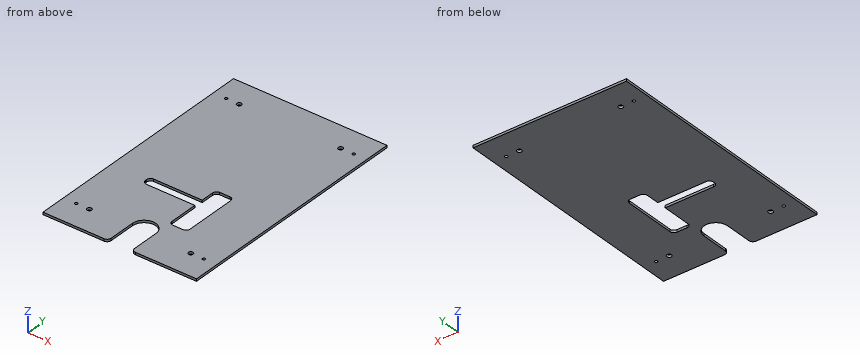
from build123d import *

# Parameters (mm, degrees)
ESQUISSE1_W             = 196
ESQUISSE1_H             = 309
ESQUISSE1_R             = 1.75
ESQUISSE1_R_2           = 3
BOSS_EXTRU_1_DEPTH      = 3
ENL_V_MAT_EXTRU_1_REACH = 5
CONG_1_R                = 5
ENL_V_MAT_EXTRU_2_DEPTH = 4
CONG_2_R                = 5


with BuildPart() as part:
    # Esquisse1 → Boss.-Extru.1 (new body)
    with BuildSketch(Plane.XY):
        Rectangle(ESQUISSE1_W, ESQUISSE1_H)
        with Locations((-81.5, 121.5)):
            Circle(ESQUISSE1_R, mode=Mode.SUBTRACT)
        with Locations((81.5, 121.5)):
            Circle(ESQUISSE1_R, mode=Mode.SUBTRACT)
        with Locations((81.5, -121.5)):
            Circle(ESQUISSE1_R, mode=Mode.SUBTRACT)
        with Locations((-81.5, -121.5)):
            Circle(ESQUISSE1_R, mode=Mode.SUBTRACT)
        with Locations((64.75, 121.5)):
            Circle(ESQUISSE1_R_2, mode=Mode.SUBTRACT)
        with Locations((-64.75, 121.5)):
            Circle(ESQUISSE1_R_2, mode=Mode.SUBTRACT)
        with Locations((-64.75, -121.5)):
            Circle(ESQUISSE1_R_2, mode=Mode.SUBTRACT)
        with Locations((64.75, -121.5)):
            Circle(ESQUISSE1_R_2, mode=Mode.SUBTRACT)
    extrude(amount=BOSS_EXTRU_1_DEPTH)

    # Esquisse2 → Enlèv. mat.-Extru.1 (cut, up to next)
    with BuildSketch(Plane.XY.offset(3), mode=Mode.PRIVATE) as enl_v_mat_extru_1_sk1:
        with BuildLine():
            Line((-15, -154.5), (-15, -115))
            ThreePointArc((-15, -115), (0, -100), (15, -115))
            Line((15, -115), (15, -154.5))
            ThreePointArc((15, -154.5), (0, -169.5), (-15, -154.5))
        make_face()
    enl_v_mat_extru_1_tool1 = extrude(enl_v_mat_extru_1_sk1.sketch, amount=-ENL_V_MAT_EXTRU_1_REACH, mode=Mode.PRIVATE) & part.part
    add(enl_v_mat_extru_1_tool1.solids().sort_by_distance((0, -134.75, 3))[0], mode=Mode.SUBTRACT)

    # Congé1
    cong_1_edges = [part.edges().sort_by_distance(p)[0] for p in [
        (-15, -154.5, 1.5),
        (15, -154.5, 1.5),
    ]]
    fillet(cong_1_edges, radius=CONG_1_R)

    # Esquisse3 → Enlèv. mat.-Extru.2 (cut, through all)
    with BuildSketch(Plane.XY.offset(3)):
        Polygon((-53, -38.5), (14, -38.5), (14, -16.5), (37, -16.5), (37, -92.5), (14, -92.5), (14, -50.5), (-53, -50.5), align=None)
    extrude(amount=-ENL_V_MAT_EXTRU_2_DEPTH, mode=Mode.SUBTRACT)

    # Congé2
    cong_2_edges = [part.edges().sort_by_distance(p)[0] for p in [
        (-53, -50.5, 1.5),
        (-53, -38.5, 1.5),
        (14, -16.5, 1.5),
        (37, -16.5, 1.5),
        (37, -92.5, 1.5),
        (14, -92.5, 1.5),
    ]]
    fillet(cong_2_edges, radius=CONG_2_R)


solid = part.part
The listing builds one solid part. Answer for the finished solid, in the listing's coordinates (mm). Round coordinates to 2 decimals unless told otherwise and drop trailing zeros. Order: outer loops, then holes, each group sorted by start corner. A loop starts at its lowest first (then second) coordinate and runs counter-clockwise, first axis right, second up. Notation, with made-up numbers: M 17.5,89 L 44.5,89 A25 cw 44.5,119 Z; hole C 58,83.5 d3. An arc over 180 degrees is marked long. Answer in a Markdown table with one row per item. Add a question column.
1) The part is cut by section A-A on x = 0. Determine the outline of the cut face in (y, z), plus the area to 4 significant figures.
2) The part is cut by section B-B on z = 1.25. Count the separate pieces of the cut face and the enclosed holes in it, plus the area to 3 significant figures.
3) Consider line 1 along Y through (x, z) = (64.75, 1.9); line 2 along Y through (x, z) = (81.5, 0.8); line 3 along X through (y, z) = (-57, 1). Determine where each line is inside the solid, lowest interval first. Write a range as from..to.
Findings below:
| question | item | result |
|---|---|---|
| 1 | outline | M -100,0 L -50.5,0 L -50.5,3 L -100,3 Z; M -38.5,0 L 154.5,0 L 154.5,3 L -38.5,3 Z |
| 1 | area | 727.5 mm² |
| 2 | separate pieces | 1 |
| 2 | enclosed holes | 9 |
| 2 | area | 56,300 mm² |
| 3 | line 1 | y = -154.5..-124.5, -118.5..118.5, 124.5..154.5 |
| 3 | line 2 | y = -154.5..-123.25, -119.75..119.75, 123.25..154.5 |
| 3 | line 3 | x = -98..14, 37..98 |
